from build123d import *

# Parameters (mm, degrees)
F0_W     = 43
F0_H     = 17.5
F1_DEPTH = 1.5
F2_W     = 9.5
F2_H     = 7.5
F3_DEPTH = 3.8
F4_W     = 32
F4_H     = 11.5
F5_DEPTH = 3
F6_W     = 39
F6_H     = 13.5
F7_DEPTH = 2
F8_R     = 2.4
F9_DEPTH = 7.5
F10_R    = 2.4


with BuildPart() as f1:
    # F0 (on Top) → F1 (new body)
    with BuildSketch(Plane.XY):
        Rectangle(F0_W, F0_H)
    extrude(amount=F1_DEPTH)

    # F2 (on face) → F3 (join)
    with BuildSketch(Plane.XY.offset(1.5)):
        with Locations((19.05, 0)):
            Rectangle(F2_W, F2_H)
    extrude(amount=F3_DEPTH)

    # F4 (on face) → F5 (join)
    with BuildSketch(Plane.XY.offset(1.5)):
        with Locations((-2.5, 0)):
            Rectangle(F4_W, F4_H)
    extrude(amount=F5_DEPTH)

    # F6 (on face) → F7 (join)
    with BuildSketch(Plane(origin=(0, 0, 0), x_dir=(1, 0, 0), z_dir=(0, 0, -1))):
        Rectangle(F6_W, F6_H)
    extrude(amount=F7_DEPTH)

    # F8 (on face) → F9 (join)
    with BuildSketch(Plane.XY.offset(4.5)):
        with Locations((5.8, 0)):
            Circle(F8_R)
    extrude(amount=F9_DEPTH)

    # F10
    f10_edges = [f1.edges().sort_by_distance(p)[0] for p in [
        (3.4, 0, 12),
    ]]
    fillet(f10_edges, radius=F10_R)


solid = f1.part
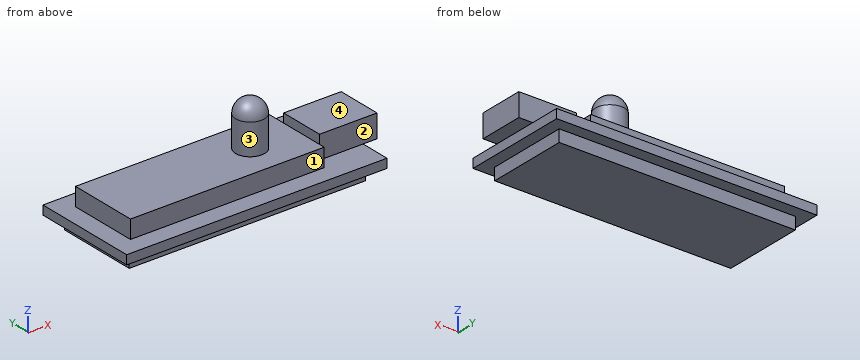
Source: CAD feature listing. Evaluate the final solid. Frame: model axes, mm. Face numbers are marked on the shaded views. A direction names the side the tool comes from. Give positions to 0.01 mm unless a question says otherwise; leave off trailing zeros. Write each loop counter-clockwise with the first axis right and the second up, starting at its lowest first coordinate (ties: lowest second). Pieces come first, ordered by that corner, then holes. Notation, with made-up numbers: M 18.25,-40 L 48.25,-40 A32 cw 48.25,-8 Z; hole C 57,1 d10. An arc over 180 degrees is marked long. Answer as a JSON object with one key per item and string values.
Q1. Cut plane B-B, the plane y = 4.5. Return the cut outline in (x, z), then the cut area to 4 significant figures.
Geometry check:
{"outline": "M -21.5,0 L -19.5,0 L -19.5,-2 L 19.5,-2 L 19.5,0 L 21.5,0 L 21.5,1.5 L 13.5,1.5 L 13.5,4.5 L -18.5,4.5 L -18.5,1.5 L -21.5,1.5 Z", "area": "238.5 mm^2"}
Q2. Cut plane A-A, the plane z = 3. Return the cut outline in (x, y).
Geometry check:
{"outline": "M -18.5,-5.75 L 13.5,-5.75 L 13.5,5.75 L -18.5,5.75 Z; M 14.3,-3.75 L 23.8,-3.75 L 23.8,3.75 L 14.3,3.75 Z"}
Q3. Contact query for flat-ended pins moving along their axis: P1, Ø1.2, axis at y = -1.5, z = 0.5, coming from the +X side; P2, Ø3, axis at x = -15, z = 4, coming from the -Y side; P3, Ø3, axis at x = 18, y = -2.5, coming from the +Z side; P4, Ø8, axis at y = 1.5, z = 8.5, coming from the +X side. Output: stop coordinate, or through.
Geometry check:
{"P1": "stops at x = 21.5", "P2": "stops at y = -5.75", "P3": "stops at z = 5.3", "P4": "stops at x = 23.8"}
Q4. Cut plane C-C, the plane x = 5.8. Return the cut outline in (y, z).
Geometry check:
{"outline": "M -8.75,0 L -6.75,0 L -6.75,-2 L 6.75,-2 L 6.75,0 L 8.75,0 L 8.75,1.5 L 5.75,1.5 L 5.75,4.5 L 2.4,4.5 L 2.4,9.6 A2.4 ccw -2.4,9.6 L -2.4,4.5 L -5.75,4.5 L -5.75,1.5 L -8.75,1.5 Z"}
Q5. Cut plane D-D, the plane y = 0. Return the cut outline in (x, z), then the cut area to 3 significant figures.
Geometry check:
{"outline": "M -21.5,0 L -19.5,0 L -19.5,-2 L 19.5,-2 L 19.5,0 L 21.5,0 L 21.5,1.5 L 23.8,1.5 L 23.8,5.3 L 14.3,5.3 L 14.3,1.5 L 13.5,1.5 L 13.5,4.5 L 8.2,4.5 L 8.2,9.6 A2.4 ccw 3.4,9.6 L 3.4,4.5 L -18.5,4.5 L -18.5,1.5 L -21.5,1.5 Z", "area": "308 mm^2"}
Q6. Access query for the marked faces 1, 2, 3 and 4. Directions: +Z, -Z, +X, -X, +Y, -Y. A direction counts if a zero-diameter tool reaches every point of the face in a straight line with its end or side. Return the directions, or none.
Geometry check:
{"face 1": "+Z, +X, -X, -Y", "face 2": "+Z, +X, -Y", "face 3": "+Z", "face 4": "+Z, +X, +Y, -Y"}
Q7. Ray query, line 1 along X through (y, z) = (2.75, 3.5); line 2 along Z through (x, y) = (-13.5, 5); line 3 along X through (y, z) = (-3, -1.25). Return the intervals inside material, ascending.
Geometry check:
{"line 1": "x = -18.5 to 13.5, 14.3 to 23.8", "line 2": "z = -2 to 4.5", "line 3": "x = -19.5 to 19.5"}
